from build123d import *

# Parameters (mm, degrees)
F0_W     = 136.419938
F0_H     = 104.761296
F0_R     = 7.008527
F1_DEPTH = 25.4


with BuildPart() as f1:
    # F0 (on Top) → F1 (new body)
    with BuildSketch(Plane.XY):
        Rectangle(F0_W, F0_H)
        with Locations((-54.395288, -37.346224)):
            Circle(F0_R, mode=Mode.SUBTRACT)
        with Locations((-39.155288, -37.346224)):
            Circle(F0_R, mode=Mode.SUBTRACT)
        with Locations((-23.915288, -37.346224)):
            Circle(F0_R, mode=Mode.SUBTRACT)
        with Locations((-8.675288, -37.346224)):
            Circle(F0_R, mode=Mode.SUBTRACT)
        with Locations((-54.395288, -22.106224)):
            Circle(F0_R, mode=Mode.SUBTRACT)
        with Locations((-39.155288, -22.106224)):
            Circle(F0_R, mode=Mode.SUBTRACT)
        with Locations((-54.395288, -6.866224)):
            Circle(F0_R, mode=Mode.SUBTRACT)
        with Locations((-39.155288, -6.866224)):
            Circle(F0_R, mode=Mode.SUBTRACT)
        with Locations((-23.915288, -22.106224)):
            Circle(F0_R, mode=Mode.SUBTRACT)
        with Locations((-8.675288, -22.106224)):
            Circle(F0_R, mode=Mode.SUBTRACT)
        with Locations((-23.915288, -6.866224)):
            Circle(F0_R, mode=Mode.SUBTRACT)
        with Locations((-8.675288, -6.866224)):
            Circle(F0_R, mode=Mode.SUBTRACT)
        with Locations((6.564712, -37.346224)):
            Circle(F0_R, mode=Mode.SUBTRACT)
        with Locations((21.804712, -37.346224)):
            Circle(F0_R, mode=Mode.SUBTRACT)
        with Locations((37.044712, -37.346224)):
            Circle(F0_R, mode=Mode.SUBTRACT)
        with Locations((52.284712, -37.346224)):
            Circle(F0_R, mode=Mode.SUBTRACT)
        with Locations((6.564712, -22.106224)):
            Circle(F0_R, mode=Mode.SUBTRACT)
        with Locations((21.804712, -22.106224)):
            Circle(F0_R, mode=Mode.SUBTRACT)
        with Locations((6.564712, -6.866224)):
            Circle(F0_R, mode=Mode.SUBTRACT)
        with Locations((21.804712, -6.866224)):
            Circle(F0_R, mode=Mode.SUBTRACT)
        with Locations((37.044712, -22.106224)):
            Circle(F0_R, mode=Mode.SUBTRACT)
        with Locations((52.284712, -22.106224)):
            Circle(F0_R, mode=Mode.SUBTRACT)
        with Locations((37.044712, -6.866224)):
            Circle(F0_R, mode=Mode.SUBTRACT)
        with Locations((52.284712, -6.866224)):
            Circle(F0_R, mode=Mode.SUBTRACT)
        with Locations((-54.395288, 8.373776)):
            Circle(F0_R, mode=Mode.SUBTRACT)
        with Locations((-39.155288, 8.373776)):
            Circle(F0_R, mode=Mode.SUBTRACT)
        with Locations((-54.395288, 23.613776)):
            Circle(F0_R, mode=Mode.SUBTRACT)
        with Locations((-39.155288, 23.613776)):
            Circle(F0_R, mode=Mode.SUBTRACT)
        with Locations((-23.915288, 8.373776)):
            Circle(F0_R, mode=Mode.SUBTRACT)
        with Locations((-8.675288, 8.373776)):
            Circle(F0_R, mode=Mode.SUBTRACT)
        with Locations((-23.915288, 23.613776)):
            Circle(F0_R, mode=Mode.SUBTRACT)
        with Locations((-8.675288, 23.613776)):
            Circle(F0_R, mode=Mode.SUBTRACT)
        with Locations((-54.395288, 38.853776)):
            Circle(F0_R, mode=Mode.SUBTRACT)
        with Locations((-39.155288, 38.853776)):
            Circle(F0_R, mode=Mode.SUBTRACT)
        with Locations((-23.915288, 38.853776)):
            Circle(F0_R, mode=Mode.SUBTRACT)
        with Locations((-8.675288, 38.853776)):
            Circle(F0_R, mode=Mode.SUBTRACT)
        with Locations((6.564712, 8.373776)):
            Circle(F0_R, mode=Mode.SUBTRACT)
        with Locations((21.804712, 8.373776)):
            Circle(F0_R, mode=Mode.SUBTRACT)
        with Locations((6.564712, 23.613776)):
            Circle(F0_R, mode=Mode.SUBTRACT)
        with Locations((21.804712, 23.613776)):
            Circle(F0_R, mode=Mode.SUBTRACT)
        with Locations((37.044712, 8.373776)):
            Circle(F0_R, mode=Mode.SUBTRACT)
        with Locations((52.284712, 8.373776)):
            Circle(F0_R, mode=Mode.SUBTRACT)
        with Locations((37.044712, 23.613776)):
            Circle(F0_R, mode=Mode.SUBTRACT)
        with Locations((52.284712, 23.613776)):
            Circle(F0_R, mode=Mode.SUBTRACT)
        with Locations((6.564712, 38.853776)):
            Circle(F0_R, mode=Mode.SUBTRACT)
        with Locations((21.804712, 38.853776)):
            Circle(F0_R, mode=Mode.SUBTRACT)
        with Locations((37.044712, 38.853776)):
            Circle(F0_R, mode=Mode.SUBTRACT)
        with Locations((52.284712, 38.853776)):
            Circle(F0_R, mode=Mode.SUBTRACT)
    extrude(amount=F1_DEPTH)


solid = f1.part
Design review of the part built by this model. Coordinates are the model's own, in mm. Round coordinates to 2 decimals unless told otherwise and drop trailing zeros. Write each loop counter-clockwise with the first axis right and the second up, starting at its lowest first coordinate (ties: lowest second). Pieces come first, ordered by that corner, then holes. Notation, with made-up numbers: M 77.25,-35.5 L 99.25,-35.5 A30 cw 99.25,-13.5 Z; hole C 24,-22.5 d4. An arc over 180 degrees is marked long. One line per item, written item: value. Start each with the question number.
1. Take a section at C-C on x = -50. State the section outline as (y, z) points.
2. Take a section at B-B on y = 19. State how many separate pieces and enclosed holes the cut face has, then the cut area to 3 significant figures.
3. Draft analysis for pull direction X (two halves, no side actions). For faces 1 (the face through (-1, -52.381, 13)), 2 (the face through (5.652, 30.563, 12.522)), 3 (the face through (43.5, -9.6, 12.5)), 4 (the face through (-68.21, -1, 13)), state which applies: pulls with the +X half, pulls with the -X half, needs draft (parallel to the pull), parting line crosses it, or undercut.
4. Take a section at A-A on x = -9.5. State the section outline as (y, z) points, then the cut area to 3 significant figures.
5. Clearance check with a flat-ended pin moving along its axis: P1, Ø8.5, axis at x = 52.28, y = 38.85, coming from the +Z side. State where the tip first meets the part, or that it passes through.
Computed:
1. outline: M -52.38,0 L -42.81,0 L -42.81,25.4 L -52.38,25.4 Z; M -31.89,0 L -27.57,0 L -27.57,25.4 L -31.89,25.4 Z; M -16.65,0 L -12.33,0 L -12.33,25.4 L -16.65,25.4 Z; M -1.41,0 L 2.91,0 L 2.91,25.4 L -1.41,25.4 Z; M 13.83,0 L 18.15,0 L 18.15,25.4 L 13.83,25.4 Z; M 29.07,0 L 33.39,0 L 33.39,25.4 L 29.07,25.4 Z; M 44.31,0 L 52.38,0 L 52.38,25.4 L 44.31,25.4 Z
2. separate pieces: 9
2. enclosed holes: 0
2. area: 1,320 mm²
3. face 1: needs draft
3. face 2: undercut
3. face 3: undercut
3. face 4: pulls with the -X half
4. outline: M -52.38,0 L -44.31,0 L -44.31,25.4 L -52.38,25.4 Z; M -30.39,0 L -29.07,0 L -29.07,25.4 L -30.39,25.4 Z; M -15.15,0 L -13.83,0 L -13.83,25.4 L -15.15,25.4 Z; M 0.09,0 L 1.41,0 L 1.41,25.4 L 0.09,25.4 Z; M 15.33,0 L 16.65,0 L 16.65,25.4 L 15.33,25.4 Z; M 30.57,0 L 31.89,0 L 31.89,25.4 L 30.57,25.4 Z; M 45.81,0 L 52.38,0 L 52.38,25.4 L 45.81,25.4 Z
4. area: 540 mm²
5. P1: passes through
